```python
from build123d import *

# Parameters (mm, degrees)
F0_W     = 76.031186
F0_H     = 76.254733
F1_DEPTH = 16.889574
F2_R     = 4.608742
F3_DEPTH = 1.204457


with BuildPart() as f1:
    # F0 (on Front) → F1 (new body)
    with BuildSketch(Plane.XZ):
        with Locations((-38.015593, 38.127367)):
            Rectangle(F0_W, F0_H)
    extrude(amount=F1_DEPTH)

    # F2 (on face) → F3 (join)
    with BuildSketch(Plane(origin=(-76.031186, 0, 0), x_dir=(0, -1, 0), z_dir=(-1, 0, 0))):
        with Locations((8.180324, 60.1198)):
            Circle(F2_R)
    extrude(amount=F3_DEPTH)


solid = f1.part
```
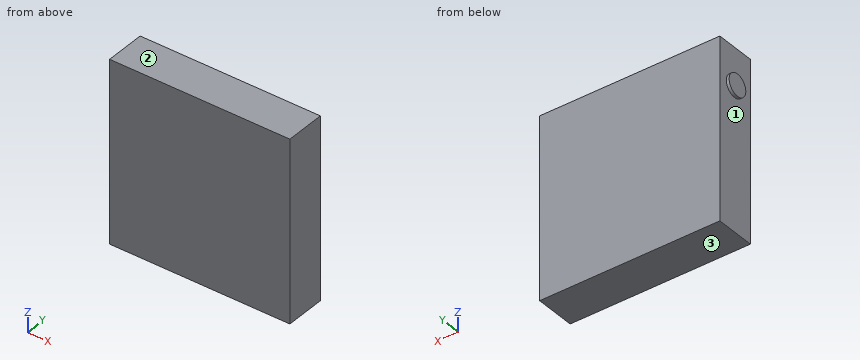
Geometry: final body of the model. Coordinates: model frame, mm. Face numbers are marked on the shaded views. Coordinates: 2 decimals unless noted, no trailing zeros. Order: outer loops, then holes, each group sorted by start corner. A loop starts at its lowest first (then second) coordinate and runs counter-clockwise, first axis right, second up. Notation, with made-up numbers: M 76.25,26 L 97.25,26 A31 ccw 97.25,62 Z; hole C -5,-16 d9. An arc over 180 degrees is marked long. Answer as CSV lines item,"result".
Q1. Section A-A on y = -1. Return the cut outline in (x, z).
Answers:
outline,"M -76.03,0 L 0,0 L 0,76.25 L -76.03,76.25 Z"
Q2. Draft query along Z for the marked faces 1, 2 and 3. Return one class per face: pulls with the +Z half, pulls with the -Z half, needs draft (parallel to the pull), parting line crosses it, or undercut.
Answers:
face 1,"needs draft"
face 2,"pulls with the +Z half"
face 3,"pulls with the -Z half"
Q3. Section B-B on z = 42.5. Return the cut outline in (x, y).
Answers:
outline,"M -76.03,-16.89 L 0,-16.89 L 0,0 L -76.03,0 Z"
Q4. First-contact query: P1, Ø6, axis at x = -68, z = 21, coming from the +Y side. Flat tip, straight axial feed; report the tip coordinate or a pass-through.
Answers:
P1,"stops at y = 0"
Q5. Line query: probe 1 along X at (y, z) = (-3, 64.5). Output: solid intervals per line, ascending. Write a range as [from, to].
Answers:
probe 1,"x = [-76.03, 0]"
